```python
from build123d import *

# Parameters (mm, degrees)
SKETCH1_R           = 1.675
BOSS_EXTRUDE1_DEPTH = 8.35
SKETCH2_R           = 1.65
BOSS_EXTRUDE2_DEPTH = 24.75
BOSS_EXTRUDE3_DEPTH = 20.8
CUT_EXTRUDE1_DEPTH  = 50.573909469
CUT_EXTRUDE2_DEPTH  = 53.287713662
SKETCH6_R           = 1.675
CUT_EXTRUDE3_DEPTH  = 10
SKETCH7_R           = 1.25
CUT_EXTRUDE4_DEPTH  = 53.287713662
CUT_EXTRUDE5_DEPTH  = 5.8
SKETCH9_W           = 12.95
SKETCH9_H           = 2.348780669
BOSS_EXTRUDE4_DEPTH = 3.24
BOSS_EXTRUDE5_DEPTH = 28.2
FILLET1_R           = 2.5
SKETCH11_R          = 1.75
CUT_EXTRUDE6_DEPTH  = 6.411671601
CUT_EXTRUDE7_DEPTH  = 3.13
CUT_EXTRUDE8_REACH  = 61.109
SKETCH13_W          = 15.68
SKETCH13_H          = 5


with BuildPart() as part:
    # Sketch1 → Boss-Extrude1 (new body)
    with BuildSketch(Plane(origin=(0, 0, 0), x_dir=(1, 0, 0), z_dir=(0, 1, 0))):
        with BuildLine():
            Line((28.2, 0), (0, 0))
            Line((0, 0), (0, -24.75))
            Line((0, -24.75), (12.95, -24.75))
            ThreePointArc((12.95, -24.75), (14.711852404, -28.091688283), (18.464508929, -28.52593877))
            Line((18.464508929, -28.52593877), (28.2, -24.75))
            Line((28.2, -24.75), (28.2, 0))
        make_face()
        with Locations(Location((17, -24.75, 0), (0, 0, 270))):
            Circle(SKETCH1_R, mode=Mode.SUBTRACT)
        with Locations(Location((17, -9.75, 0), (0, 0, 270))):
            Circle(SKETCH1_R, mode=Mode.SUBTRACT)
    extrude(amount=BOSS_EXTRUDE1_DEPTH)

    # Sketch2 → Boss-Extrude2 (add)
    with BuildSketch(Plane(origin=(0, 0, 0), x_dir=(-1, 0, 0), z_dir=(0, 0, -1))):
        with BuildLine():
            Line((-32.3, 2.75), (-28.2, 2.75))
            Line((-28.2, 2.75), (-28.2, 8.35))
            Line((-28.2, 8.35), (-28.484243194, 8.35))
            ThreePointArc((-28.484243194, 8.35), (-35.688214869, 9.158679276), (-32.3, 2.75))
        make_face()
        with Locations((-32.3, 6.85)):
            Circle(SKETCH2_R, mode=Mode.SUBTRACT)
    extrude(amount=-BOSS_EXTRUDE2_DEPTH)

    # Sketch3 → Boss-Extrude3 (add)
    with BuildSketch(Plane(origin=(0, 8.35, 0), x_dir=(1, 0, 0), z_dir=(0, 1, 0))):
        with BuildLine():
            Line((27.9, -5.15), (0, -5.15))
            Line((0, -5.15), (0, -7.75))
            Line((0, -7.75), (13.5, -7.75))
            Line((13.5, -7.75), (13.5, -15.8))
            ThreePointArc((13.5, -15.8), (17, -19.3), (20.5, -15.8))
            Line((20.5, -15.8), (20.5, -12.2))
            Line((20.5, -12.2), (27.9, -12.2))
            Line((27.9, -12.2), (27.9, -5.15))
        make_face()
    extrude(amount=BOSS_EXTRUDE3_DEPTH)

    # Sketch4 → Cut-Extrude1 (cut, through all)
    with BuildSketch(Plane(origin=(27.9, 0, 0), x_dir=(0, 0, -1), z_dir=(1, 0, 0))):
        Polygon((-5.15, 29.15), (-19.3, 20.980493691), (-19.3, 29.15), align=None)
    extrude(amount=-CUT_EXTRUDE1_DEPTH, mode=Mode.SUBTRACT)

    # Sketch5 → Cut-Extrude2 (cut, through all)
    with BuildSketch(Plane(origin=(0, 0, 5.15), x_dir=(-1, 0, 0), z_dir=(0, 0, -1))):
        with BuildLine():
            Line((-6, 21.65), (0, 21.65))
            Line((0, 21.65), (0, 29.15))
            Line((0, 29.15), (-13.5, 29.15))
            ThreePointArc((-13.5, 29.15), (-11.303300859, 23.846699141), (-6, 21.65))
        make_face()
    extrude(amount=-CUT_EXTRUDE2_DEPTH, mode=Mode.SUBTRACT)

    # Sketch6 → Cut-Extrude3 (cut)
    with BuildSketch(Plane(origin=(0, 24.092515415, 13.90982026), x_dir=(1, 0, 0), z_dir=(0, 0.8660254037844362, 0.5000000000000046))):
        with Locations(Location((17, -2.182591563, 0), (0, 0, 270))):
            Circle(SKETCH6_R)
    extrude(amount=-CUT_EXTRUDE3_DEPTH, mode=Mode.SUBTRACT)

    # Sketch7 → Cut-Extrude4 (cut, through all)
    with BuildSketch(Plane(origin=(0, 0, 5.15), x_dir=(-1, 0, 0), z_dir=(0, 0, -1))):
        with Locations((-24, 18.5)):
            Circle(SKETCH7_R)
    extrude(amount=-CUT_EXTRUDE4_DEPTH, mode=Mode.SUBTRACT)

    # Sketch8 → Cut-Extrude5 (cut)
    with BuildSketch(Plane(origin=(0, 8.35, 0), x_dir=(1, 0, 0), z_dir=(0, 1, 0))):
        with BuildLine():
            Line((13, -10.35), (13, -17.642893219))
            ThreePointArc((13, -17.642893219), (12.691341716, -18.104832985), (12.146446609, -17.996446609))
            Line((12.146446609, -17.996446609), (5.353553391, -11.203553391))
            ThreePointArc((5.353553391, -11.203553391), (5.245167015, -10.658658284), (5.707106781, -10.35))
            Line((5.707106781, -10.35), (13, -10.35))
        make_face()
        with BuildLine():
            Line((1.887867966, -11.131980515), (12.803553391, -22.04766594))
            ThreePointArc((12.803553391, -22.04766594), (12.911939766, -22.209877615), (12.95, -22.401219331))
            Line((12.95, -22.401219331), (12.95, -24.75))
            Line((12.95, -24.75), (0, -24.75))
            Line((0, -24.75), (0, -10.35))
            ThreePointArc((0, -10.35), (1.021706781, -10.553230114), (1.887867966, -11.131980515))
        make_face()
    extrude(amount=-CUT_EXTRUDE5_DEPTH, mode=Mode.SUBTRACT)

    # Sketch9 → Boss-Extrude4 (add)
    with BuildSketch(Plane(origin=(0, 2.55, 0), x_dir=(1, 0, 0), z_dir=(0, 1, 0))):
        with Locations((6.475, -23.575609666)):
            Rectangle(SKETCH9_W, SKETCH9_H)
    extrude(amount=BOSS_EXTRUDE4_DEPTH)

    # Sketch10 → Boss-Extrude5 (add)
    with BuildSketch(Plane.ZY):
        Polygon((0, 8.35), (-8.569597977, 13.297659699), (-11.775433778, 7.744989211), (-3.11517974, 2.744989211), (-4.7, 0), (0, 0), align=None)
    extrude(amount=-BOSS_EXTRUDE5_DEPTH)

    # Fillet1
    fillet1_edges = [part.edges().sort_by_distance(p)[0] for p in [
        (28.2, 10.521324455, -10.172515877),
    ]]
    fillet(fillet1_edges, radius=FILLET1_R)

    # Sketch11 → Cut-Extrude6 (cut)
    with BuildSketch(Plane(origin=(0, 0.709829513, 0.40982026), x_dir=(1, 0, 0), z_dir=(0, -0.8660254037844389, -0.4999999999999994))):
        with Locations((0, -10.070319398)):
            Circle(SKETCH11_R)
        with Locations(Location((22, -10.070319398, 0), (0, 0, 270))):
            Circle(SKETCH11_R)
    extrude(amount=-CUT_EXTRUDE6_DEPTH, mode=Mode.SUBTRACT)

    # Sketch12 → Cut-Extrude7 (cut)
    with BuildSketch(Plane(origin=(0, 0.709829513, 0.40982026), x_dir=(1, 0, 0), z_dir=(0, -0.8660254037844389, -0.4999999999999994))):
        with BuildLine():
            Line((19.935417718, -6.470319398), (2.064582282, -6.470319398))
            ThreePointArc((2.064582282, -6.470319398), (3.929893445, -8.736738687), (3.8291644, -11.670319398))
            Line((3.8291644, -11.670319398), (18.1708356, -11.670319398))
            ThreePointArc((18.1708356, -11.670319398), (18.070106555, -8.736738687), (19.935417718, -6.470319398))
        make_face()
    extrude(amount=-CUT_EXTRUDE7_DEPTH, mode=Mode.SUBTRACT)

    # Cut-Extrude8: up to this plane
    cut_extrude8_end = Plane(origin=(0, 29.15, 5.15), z_dir=(0, 0, -1))
    # Sketch13 → Cut-Extrude8 (cut, up to the surface)
    with BuildSketch(Plane(origin=(0, 7.035159699, -12.185254038), x_dir=(-1, 0, 0), z_dir=(0, 0.4999999999999996, -0.8660254037844388)), mode=Mode.PRIVATE) as cut_extrude8_sk1:
        with Locations((-10.84, 9.731312122)):
            Rectangle(SKETCH13_W, SKETCH13_H)
    cut_extrude8_tool1 = split(extrude(cut_extrude8_sk1.sketch, amount=-CUT_EXTRUDE8_REACH, mode=Mode.PRIVATE), bisect_by=cut_extrude8_end, keep=Keep.BOTH, mode=Mode.PRIVATE)
    add(cut_extrude8_tool1.solids().sort_by_distance((10.84, 15.462723, -7.319598))[0], mode=Mode.SUBTRACT)

    # Mirror1: part across plane


with BuildPart() as part_1:
    add(part.part)
    add(part.part.mirror(Plane(origin=(0, 8.35, 24.75), x_dir=(0, 0, 1), z_dir=(1, 0, 0))))


solid = part_1.part
```
Geometry check sheet. Reference: the model listing, model coordinates, mm. A direction names the side the tool comes from. Round coordinates to 2 decimals unless told otherwise and drop trailing zeros. Order: outer loops, then holes, each group sorted by start corner. A loop starts at its lowest first (then second) coordinate and runs counter-clockwise, first axis right, second up. Notation, with made-up numbers: (16.25, -15) - (45.25, -15) arc R19 ccw to (45.25, -6) - close; hole circle Ø4 at (28.25, 18.25). An arc over 180 degrees is marked (long way). Use a Markdown table: item, result. Add a question column.
(1) Material ranges on line 1 along X through (y, z) = (14, 14.5); line 2 along X through (y, z) = (26, 9); line 3 along X through (y, z) = (10.5, 11.5), recorded low to high. Write a range as [from, to].
(2) Sectioned sample at B-B, the plane z = 20.5. Enter the section's corners in (x, y), and give its area (3 significant figures).
(3) Depth check by flat-ended pin: pin 1 (5 mm diameter, centred on y = 4, z = 16, fed in from -X); pin 2 (1 mm diameter, centred on x = -23, y = 18.5, fed in from +Z); pin 3 (1.7 mm diameter, centred on x = -10.5, y = 4.5, fed in from +Z); pin 4 (6 mm diameter, centred on y = 6, z = 20.5, fed in from +X). Enter the tip coordinate at first touch or a pass-through.
(4) Tool access check on faces 4 (the cylindrical face through (11.361, 23.905, 6.432)), 5 (the cylindrical face through (3.916, 6.395, -6.35)), 6 (the cylindrical face through (-16.9, 15.6, 19.3)), 7 (the flat face through (3, 7, 3)). Record the directions out of +Z, -Z, +X, -X, +Y, -Y that give a thin tool (end or side, any length) a straight path to the whole face; none if there is none.
(5) Release check for a two-part mould opening along X. For faces 1 (the flat face through (30.5, 6.9, 0)), 2 (the cylindrical face through (-35.617, 9.26, 12.202)), 3 (the flat face through (23.264, 4.117, 26.664)) record: pulls with the +X half, pulls with the -X half, needs draft (parallel to the pull), parting line crosses it, or undercut.
Answers below:
| question | item | result |
|---|---|---|
| 1 | line 1 | [-20.5, -13.5], [13.5, 20.5] |
| 1 | line 2 | [-27.9, -13.5], [13.5, 27.9] |
| 1 | line 3 | [-34.17, -30.43], [-27.9, -13.5], [13.5, 27.9], [30.43, 34.17] |
| 2 | outline | (-32.3, 2.75) - (-28.2, 2.75) - (-28.2, 0) - (28.2, 0) - (28.2, 2.75) - (32.3, 2.75) arc R4.1 ccw (long way) to (28.48, 8.35) - (11.26, 8.35) - (11.26, 2.55) - (-11.26, 2.55) - (-11.26, 8.35) - (-28.48, 8.35) arc R4.1 ccw (long way) to start; hole circle Ø3.3 at (-32.3, 6.85); hole circle Ø3.3 at (32.3, 6.85) |
| 2 | area | 436 mm² |
| 3 | pin 1 | x = -36.39 |
| 3 | pin 2 | z = 12.2 |
| 3 | pin 3 | z = 24.75 |
| 3 | pin 4 | x = 36.4 |
| 4 | face 4 | +Z, -Z, +Y |
| 4 | face 5 | none |
| 4 | face 6 | +Z, +Y |
| 4 | face 7 | +Y |
| 5 | face 1 | needs draft |
| 5 | face 2 | undercut |
| 5 | face 3 | pulls with the +X half |
